```python
from build123d import *

# Parameters (mm, degrees)
SKETCH1_W                  = 139.7
SKETCH1_H                  = 254
BASE_DEPTH                 = 5.08
SKETCH2_W                  = 139.7
SKETCH2_H                  = 254
SKETCH2_W_2                = 129.54
SKETCH2_H_2                = 243.84
WALLS_DEPTH                = 50.8
SKETCH4_W                  = 129.54
SKETCH4_H                  = 50.8
BOTTOM_CUT_DEPTH           = 139.7
SKETCH12_W                 = 20.32
SKETCH12_H                 = 10.16
SKETCH12_H_2               = 20.32
MOUNTING_STRUTS_DEPTH      = 50.8
SKETCH13_R                 = 1.778
PANEL_MOUNTING_HOLES_DEPTH = 12.7
BOSS_EXTRUDE6_START        = -48.768
SKETCH14_W                 = 20.32
SKETCH14_H                 = 10.16
BOSS_EXTRUDE6_DEPTH        = 50.8
SKETCH17_R                 = 1.778
FRONT_MOUNTING_HOLES_DEPTH = 12.7
CORNER_FILLET_R            = 2.54
SKETCH18_W                 = 20.32
SKETCH18_H                 = 13.97
INSERT_MOUNT_DEPTH         = 37.592
SKETCH19_R                 = 1.778
CUT_EXTRUDE1_DEPTH         = 12.7
SKETCH20_W                 = 57.15
SKETCH20_H                 = 114.3
ARDUINO_MOUNT_DEPTH        = 6.35
SKETCH21_R                 = 1.778
CUT_EXTRUDE2_DEPTH         = 7.62


with BuildPart() as part:
    # Sketch1 → Base (new body)
    with BuildSketch(Plane(origin=(0, 0, 0), x_dir=(1, 0, 0), z_dir=(0, 1, 0))):
        with Locations((69.85, 127)):
            Rectangle(SKETCH1_W, SKETCH1_H)
    extrude(amount=BASE_DEPTH)

    # Sketch2 → Walls (add)
    with BuildSketch(Plane(origin=(0, 5.08, 0), x_dir=(1, 0, 0), z_dir=(0, 1, 0))):
        with Locations((69.85, 127)):
            Rectangle(SKETCH2_W, SKETCH2_H)
        with Locations((69.85, 127)):
            Rectangle(SKETCH2_W_2, SKETCH2_H_2, mode=Mode.SUBTRACT)
    extrude(amount=WALLS_DEPTH)

    # Sketch4 → Bottom Cut (cut)
    with BuildSketch(Plane.XY):
        with Locations((69.85, 30.48)):
            Rectangle(SKETCH4_W, SKETCH4_H)
    extrude(amount=-BOTTOM_CUT_DEPTH, mode=Mode.SUBTRACT)

    # Sketch12 → Mounting Struts (add)
    with BuildSketch(Plane(origin=(0, 5.08, 0), x_dir=(1, 0, 0), z_dir=(0, 1, 0))):
        with Locations((124.46, 243.84)):
            Rectangle(SKETCH12_W, SKETCH12_H)
        with Locations((15.24, 243.84)):
            Rectangle(SKETCH12_W, SKETCH12_H)
        with Locations((124.46, 115.57)):
            Rectangle(SKETCH12_W, SKETCH12_H_2)
        with Locations((15.24, 115.57)):
            Rectangle(SKETCH12_W, SKETCH12_H_2)
    extrude(amount=MOUNTING_STRUTS_DEPTH)

    # Sketch13 → Panel Mounting Holes (cut)
    with BuildSketch(Plane(origin=(0, 55.88, 0), x_dir=(1, 0, 0), z_dir=(0, 1, 0))):
        with Locations((120.65, 243.713)):
            Circle(SKETCH13_R)
        with Locations((19.05, 243.713)):
            Circle(SKETCH13_R)
        with Locations((120.65, 116.713)):
            Circle(SKETCH13_R)
        with Locations((19.05, 116.713)):
            Circle(SKETCH13_R)
    extrude(amount=-PANEL_MOUNTING_HOLES_DEPTH, mode=Mode.SUBTRACT)

    # Sketch14 → Boss-Extrude6 (add)
    with BuildSketch(Plane(origin=(0, 53.848, 0), x_dir=(1, 0, 0), z_dir=(0, 1, 0)).offset(BOSS_EXTRUDE6_START)):
        with Locations((124.46, 10.16)):
            Rectangle(SKETCH14_W, SKETCH14_H)
        with Locations((15.24, 10.16)):
            Rectangle(SKETCH14_W, SKETCH14_H)
    extrude(amount=BOSS_EXTRUDE6_DEPTH)

    # Sketch17 → Front Mounting Holes (cut)
    with BuildSketch(Plane(origin=(0, 55.88, 0), x_dir=(1, 0, 0), z_dir=(0, 1, 0))):
        with Locations((129.54, 243.713)):
            Circle(SKETCH17_R)
        with Locations((10.16, 243.713)):
            Circle(SKETCH17_R)
        with Locations((10.16, 116.713)):
            Circle(SKETCH17_R)
        with Locations((129.54, 116.713)):
            Circle(SKETCH17_R)
        with Locations((129.54, 8.763)):
            Circle(SKETCH17_R)
        with Locations((10.16, 8.763)):
            Circle(SKETCH17_R)
    extrude(amount=-FRONT_MOUNTING_HOLES_DEPTH, mode=Mode.SUBTRACT)

    # Corner Fillet
    corner_fillet_edges = [part.edges().sort_by_distance(p)[0] for p in [
        (0, 27.94, -254),
        (139.7, 27.94, -254),
        (139.7, 27.94, 0),
        (0, 27.94, 0),
    ]]
    fillet(corner_fillet_edges, radius=CORNER_FILLET_R)

    # Sketch18 → Insert Mount (add)
    with BuildSketch(Plane(origin=(0, 5.08, 0), x_dir=(1, 0, 0), z_dir=(0, 1, 0))):
        with Locations((15.24, 98.425)):
            Rectangle(SKETCH18_W, SKETCH18_H)
        with Locations((124.46, 98.425)):
            Rectangle(SKETCH18_W, SKETCH18_H)
        with Locations((124.46, 22.225)):
            Rectangle(SKETCH18_W, SKETCH18_H)
        with Locations((15.24, 22.225)):
            Rectangle(SKETCH18_W, SKETCH18_H)
    extrude(amount=INSERT_MOUNT_DEPTH)

    # Sketch19 → Cut-Extrude1 (cut)
    with BuildSketch(Plane(origin=(0, 42.672, 0), x_dir=(1, 0, 0), z_dir=(0, 1, 0))):
        with Locations((12.7, 99.06)):
            Circle(SKETCH19_R)
        with Locations((127, 99.06)):
            Circle(SKETCH19_R)
        with Locations((127, 21.59)):
            Circle(SKETCH19_R)
        with Locations((12.7, 21.59)):
            Circle(SKETCH19_R)
    extrude(amount=-CUT_EXTRUDE1_DEPTH, mode=Mode.SUBTRACT)

    # Sketch20 → Arduino Mount (add)
    with BuildSketch(Plane(origin=(0, 5.08, 0), x_dir=(1, 0, 0), z_dir=(0, 1, 0))):
        with Locations((69.85, 191.77)):
            Rectangle(SKETCH20_W, SKETCH20_H)
    extrude(amount=ARDUINO_MOUNT_DEPTH)

    # Sketch21 → Cut-Extrude2 (cut)
    with BuildSketch(Plane.XY.offset(-5.08)):
        with Locations((128.27, 11.43)):
            Circle(SKETCH21_R)
        with Locations((128.27, 39.37)):
            Circle(SKETCH21_R)
        with Locations((11.43, 39.37)):
            Circle(SKETCH21_R)
        with Locations((11.43, 11.43)):
            Circle(SKETCH21_R)
    extrude(amount=-CUT_EXTRUDE2_DEPTH, mode=Mode.SUBTRACT)


solid = part.part
```
For this review, take the finished solid that the model builds, in its own axes (mm). A direction names the side the tool comes from. Give positions to 0.01 mm unless a question says otherwise; leave off trailing zeros. Loops run counter-clockwise (first coordinate to the right, second up) from the corner with the lowest first, then second, coordinate; pieces in that order, holes last. Notation, with made-up numbers: M 89.5,30 L 122.5,30 A19 cw 122.5,54 Z; hole C 53,24 d6. An arc over 180 degrees is marked long. One line per item, written item: value. Start each with the question number.
Q1. Add section A-A (z = -158). Give the boundary of the cut face in (x, y) (3 decimals).
Q2. Machinability: for faces 1 (the face through (25.4, 30, -108)), 2 (the face through (124, 30, -238.76)), 3 (the face through (139.7, 28, -125)), which of the approach directions +Z, -Z, +X, -X, +Y, -Y give a long, thin tool a straight path to every point of the face, cutting with its end or side? Answer none if there is none.
Q3. Add section C-C (x = 28). Give the boundary of the cut face in (y, z).
Q4. Add section D-D (z = -49.5). Give the boundary of the cut face in (x, y).
Q5. For L1, parallel to Z at x = 10.16, y = 50.5 (3 decimals); L2, parallel to Z at x = 127, y = 35; L3, parallel to Z at x = 15, y = 16.5, list the stretches that pass through material, from the lowest coordinate up.
Q6. Clearance check with flat-ended pins moving along their axes: pin 1 Ø1.1 at (x, z) = (9.5, -116.5) entering from +Y; pin 2 Ø6 at (x, z) = (76, -211) entering from +Y; pin 3 Ø4.5 at (x, z) = (127, -99.06) entering from +Y. State where each tip first meets the part, or that it passes through.
Q7. Add section B-B (y = 35). Count the separate pieces of the cut face and the enclosed holes in it, and give its area (3 significant figures).
Q8. Draft analysis for pull direction Z (two halves, no side actions). For faces 4 (the face through (25.4, 30, -17)), 5 (the face through (69, 28, -254)), 6 (the face through (134.62, 30, -181)), state which applies: released by +Z, released by -Z, zero draft, split by the parting line, or undercut.
Reply:
1. outline: M 0,0 L 139.7,0 L 139.7,55.88 L 134.62,55.88 L 134.62,5.08 L 98.425,5.08 L 98.425,11.43 L 41.275,11.43 L 41.275,5.08 L 5.08,5.08 L 5.08,55.88 L 0,55.88 Z
2. face 1: +Z, +Y
2. face 2: +Y
2. face 3: +Z, -Z, +X, +Y, -Y
3. outline: M 0,-254 L 55.88,-254 L 55.88,-248.92 L 5.08,-248.92 L 5.08,0 L 0,0 Z
4. outline: M 0,0 L 139.7,0 L 139.7,55.88 L 134.62,55.88 L 134.62,5.08 L 5.08,5.08 L 5.08,55.88 L 0,55.88 Z
5. L1: -254 to -245.491, -241.935 to -238.76, -125.73 to -118.491, -114.935 to -105.41, -15.24 to -10.541, -6.985 to -5.08
5. L2: -254 to -238.76, -125.73 to -100.84, -97.28 to -91.44, -29.21 to -23.37, -19.81 to -5.08
5. L3: -254 to -238.76, -125.73 to -91.44, -29.21 to -5.08
6. pin 1: y = 43.18
6. pin 2: y = 11.43
6. pin 3: y = 42.67
7. separate pieces: 1
7. enclosed holes: 4
7. area: 5,980 mm²
8. face 4: zero draft
8. face 5: released by -Z
8. face 6: undercut
